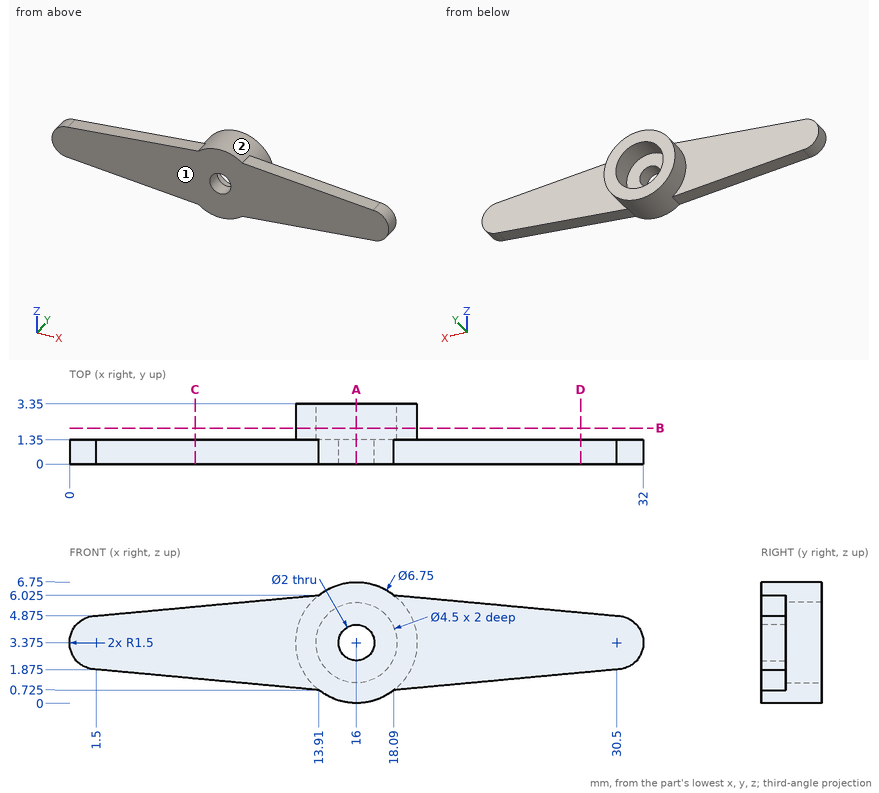
Here's the drawing with two shaded views (mm, measured from the low corner). I have some questions. A direction names the side the tool comes from. Give positions to 0.01 mm unless a question says otherwise; leave off trailing zeros. Write each loop counter-clockwise with the first axis right and the second up, starting at its lowest first coordinate (ties: lowest second). Pieces come first, ordered by that corner, then holes. Notation, with made-up numbers: (36.25, -32.5) -> (60.25, -32.5) arc R34 cw to (60.25, -2.5) -> close; hole circle Ø9 at (73, 5.25). An arc over 180 degrees is marked (long way). Use one line per item in the form item = value. Start each with the question number.
1. Will these pins go through, and if not, where does the flat tip stop? pin 1 Ø1.3 at (x, z) = (15.5, 2.5) entering from +Y; pin 2 Ø1.5 at (y, z) = (0.5, 5) entering from -X; pin 3 Ø3 at (x, z) = (16, 3.375) entering from -Y; pin 4 Ø2 at (y, z) = (2.5, 2) entering from -X.
2. On a 3-axis mill with a long thin cutter (end or side, diameter ignored), from which of +Z, -Z, +X, -X, +Y, -Y can I reach the whole of each face in a straight line? I mean the marked faces 1 and 2. Say none if no direction works.
3. Imagine slicing it at B-B on y = 2. List the corners of the cut face in (x, z) for me (3 decimals).
4. Imagine slicing it at A-A on x = 16. List the corners of the cut face in (y, z) for me (3 decimals).
5. Imagine slicing it at D-D on x = 28.5. List the corners of the cut face in (y, z) for me.
6. If I drill on L1, parallel to X at y = 2.1, z = 3.25; L2, parallel to Y at x = 17, z = 4.5; L3, parallel to X at y = 1.9, z = 2.75, over which ranges is the centre line in solid material (lowest first)?
7. Imagine slicing it at C-C on x = 7. List the corners of the cut face in (y, z) for me, plus the area to 3 significant figures.
Entries:
q1.pin_1 = 1.35
q1.pin_2 = 0.28
q1.pin_3 = 0
q1.pin_4 = 12.65
q2.face_1 = +Z, -Z, +X, -X, -Y
q2.face_2 = +Y
q3.outline = circle Ø6.75 at (16, 3.375); hole circle Ø4.5 at (16, 3.375)
q4.outline = (0, 0) -> (3.35, 0) -> (3.35, 1.125) -> (1.35, 1.125) -> (1.35, 2.375) -> (0, 2.375) -> close; (0, 4.375) -> (1.35, 4.375) -> (1.35, 5.625) -> (3.35, 5.625) -> (3.35, 6.75) -> (0, 6.75) -> close
q5.outline = (0, 1.69) -> (1.35, 1.69) -> (1.35, 5.06) -> (0, 5.06) -> close
q6.L1 = 12.63 to 13.75, 18.25 to 19.37
q6.L2 = 0 to 1.35
q6.L3 = 12.68 to 13.84, 18.16 to 19.32
q7.outline = (0, 1.37) -> (1.35, 1.37) -> (1.35, 5.38) -> (0, 5.38) -> close
q7.area = 5.43 mm²
